from build123d import *

# Parameters (mm, degrees)
SKETCH1_W           = 50.8
SKETCH1_H           = 77.5716
BOSS_EXTRUDE1_DEPTH = 19.8501
SKETCH2_R           = 3.3734375
CUT_EXTRUDE1_DEPTH  = 95.826260058
SKETCH3_R           = 3.3734375
CUT_EXTRUDE2_DEPTH  = 95.826260058


with BuildPart() as part:
    # Sketch1 → Boss-Extrude1 (new body)
    with BuildSketch(Plane(origin=(0, 0, 0), x_dir=(1, 0, 0), z_dir=(0, 1, 0))):
        with Locations((25.4, 38.7858)):
            Rectangle(SKETCH1_W, SKETCH1_H)
    extrude(amount=BOSS_EXTRUDE1_DEPTH)

    # Sketch2 → Cut-Extrude1 (cut, through all)
    with BuildSketch(Plane(origin=(0, 19.8501, 0), x_dir=(1, 0, 0), z_dir=(0, 1, 0))):
        with Locations(Location((20.574, 19.735800015, 0), (0, 0, 270))):
            Circle(SKETCH2_R)
        with Locations(Location((20.574, 57.835800015, 0), (0, 0, 270))):
            Circle(SKETCH2_R)
    extrude(amount=-CUT_EXTRUDE1_DEPTH, mode=Mode.SUBTRACT)

    # Sketch3 → Cut-Extrude2 (cut, through all)
    with BuildSketch(Plane.XY):
        with Locations((7.62, 9.92505)):
            Circle(SKETCH3_R)
        with Locations((43.18, 9.92505)):
            Circle(SKETCH3_R)
    extrude(amount=-CUT_EXTRUDE2_DEPTH, mode=Mode.SUBTRACT)


solid = part.part
Part model, mm, in its own coordinate system. Give positions to 0.01 mm unless a question says otherwise; leave off trailing zeros. Order: outer loops, then holes, each group sorted by start corner. A loop starts at its lowest first (then second) coordinate and runs counter-clockwise, first axis right, second up. Notation, with made-up numbers: (-27, 68.5) -> (9, 68.5) arc R26 cw to (9, 96.5) -> close; hole circle Ø3 at (81, -20.5). An arc over 180 degrees is marked (long way). Use one line per item in the form item = value.
(1) Saw through at B-B (y = 15.5). Write the cut outline in (x, z), then the cut area to 3 significant figures.
Solution:
outline = (0, -77.57) -> (50.8, -77.57) -> (50.8, 0) -> (0, 0) -> close; hole circle Ø6.75 at (20.57, -57.84); hole circle Ø6.75 at (20.57, -19.74)
area = 3,870 mm²
(2) Flat gauge pin, fed straight in: P1, Ø4, axis at x = 20.57, z = -19.74, coming from the +Y side. Where does the tip first touch, or does it go through?
Solution:
P1 = through
(3) Saw through at C-C (z = -12.5). Write the cut outline in (x, y).
Solution:
outline = (0, 0) -> (50.8, 0) -> (50.8, 19.85) -> (0, 19.85) -> close; hole circle Ø6.75 at (7.62, 9.93); hole circle Ø6.75 at (43.18, 9.93)
(4) Pull direction Z, two halves, no side cores. Call faces 1 (the face through (22.854, 10.064, -60.322)), 2 (the face through (25, 10, -77.572)), 3 (the face through (25, 0, -39)): +Z half, -Z half, draft (parallel to the pull), parting line (faces both ways), or undercut.
Solution:
face_1 = undercut
face_2 = -Z half
face_3 = draft
(5) Drill centre lines: line 1 (X direction, y = 8.75, z = -48); line 2 (X direction, y = 12.75, z = -48.5); line 3 (Z direction, x = 20, y = 18.75). Where is each one in solid material? Low to high. Write a range as from..to.
Solution:
line_1 = 0..4.46, 10.78..40.02, 46.34..50.8
line_2 = 0..5.78, 9.46..41.34, 45.02..50.8
line_3 = -77.57..-61.16, -54.51..-23.06, -16.41..0
(6) Saw through at A-A (x = 7.62). Write the cut outline in (y, z), then the cut area to 3 significant figures.
Solution:
outline = (0, -77.57) -> (6.55, -77.57) -> (6.55, 0) -> (0, 0) -> close; (13.3, -77.57) -> (19.85, -77.57) -> (19.85, 0) -> (13.3, 0) -> close
area = 1,020 mm²
